Autodesk Inventor part; units mm, degrees
ref_plane "YZ Plane" through (0, 0, 0) normal (1, 0, 0) x (0, 1, 0)
ref_plane "XZ Plane" through (0, 0, 0) normal (0, 1, 0) x (-1, 0, 0)
ref_plane "XY Plane" through (0, 0, 0) normal (0, 0, 1) x (1, 0, 0)
sketch "Sketch1" plane through (0, 0, 0) normal (0, 0, 1) x (1, 0, 0)
  circle A0 centre (0, 0) radius 10.75
  dimension "d0" = 21.5
extrude "Extrusion1" add sketch "Sketch1" along normal blind 48
sketch "Sketch2" plane through (0, 0, 48) normal (0, 0, 1) x (1, 0, 0)
  circle A0 centre (0, 0) radius 10.75
  circle A1 centre (0, 0) radius 5
  dimension "d3" = 10
extrude "Extrusion2" cut sketch "Sketch2" against normal blind 45
chamfer "Chamfer1" distance 0.5 angle 45 1 edges at (-5, 0, 48)
fillet "Fillet1" radius 0.5 1 edges at (-5, 0, 3)
sketch "Sketch3" plane through (0, 0, 0) normal (0, 1, 0) x (-1, 0, 0)
  line L0 (-4.5, 48) -> (4.5, 48)
  line L1 (5, 47.5) -> (-5, 47.5)
  line L2 (-5, 3.5) -> (5, 3.5)
  circle A0 centre (0, 42) radius 2
  point P0 (0, 0)
  dimension "d10" = 4
  dimension "d11" = 6
extrude "Extrusion3" cut sketch "Sketch3" along normal mid plane 15
properties part number "EIXO DAS ENGRENAGENS(11)" material "Carbon Steel"
Check sheet for the modelled part. Datum: model origin and axes. Units: mm. A direction names the side the tool comes from. Give positions to 0.01 mm unless a question says otherwise; leave off trailing zeros. Loops run counter-clockwise (first coordinate to the right, second up) from the corner with the lowest first, then second, coordinate; pieces in that order, holes last. Notation, with made-up numbers: M -1,75.25 L 39,75.25 A16 cw 39,87.25 Z; hole C 21,85.5 d8. An arc over 180 degrees is marked long. Use a Markdown table: item, result. Add a question column.
Q1. Sectioned sample at D-D, the plane z = 15. Record the cut outline in (x, y).
Q2. Sectioned sample at B-B, the plane y = 0. Record the cut outline in (x, z).
Q3. Scan lines: line 1 along X through (y, z) = (-0.25, 42); line 2 along Z through (x, y) = (0, -1.5); line 3 along Z through (x, y) = (4.75, 7.5). Record each from-to range of solid material in increasing order. Write a range as [from, to].
Q4. Sectioned sample at A-A, the plane x = 0. Record the cut outline in (y, z).
Q5. Go/stop test with flat-tipped pins: pin 1 (3 mm diameter, centred on y = 1.5, z = 33.5, fed in from +X); pin 2 (8 mm diameter, centred on x = 7, z = 19.5, fed in from +Y); pin 3 (5 mm diameter, centred on x = 0, z = 42, fed in from +Y); pin 4 (2 mm diameter, centred on x = -7.5, z = 18, fed in from -Y). Record where each tip stops, or that it passes through.
Q6. Tool access check on faces 4 (the flat face through (0, 0, 0)), 5 (the flat face through (-3, 5, 3)). Record the directions out of +Z, -Z, +X, -X, +Y, -Y that give a thin tool (end or side, any length) a straight path to the whole face; none if there is none.
Q7. Mould release check, pull along X, two halves, no side actions. Record for faces 1 (the cylindrical face through (4.77, 1.5, 25.81)), 2 (the cylindrical face through (-0.923, -0.07, 43.774)), 3 (the flat face through (0, 0, 48)): pulls with the +X half, pulls with the -X half, needs draft (parallel to the pull), parting line crosses it, or undercut.
Q8. Sectioned sample at C-C, the plane z = 42. Record the cut outline in (x, y).
Verdict:
| question | item | result |
|---|---|---|
| 1 | outline | C 0,0 d10 |
| 2 | outline | M -10.75,0 L 10.75,0 L 10.75,3 L 5.5,3 A0.5 cw 5,3.5 L 5,47.5 L 4.5,48 L -4.5,48 L -5,47.5 L -5,3.5 A0.5 cw -5.5,3 L -10.75,3 Z; hole C 0,42 d4 |
| 3 | line 1 | [-4.99, -2], [2, 4.99] |
| 3 | line 2 | [0, 40], [44, 48] |
| 3 | line 3 | [0, 3] |
| 4 | outline | M -10.75,0 L 10.75,0 L 10.75,3 L 5.5,3 A0.5 cw 5,3.5 L 5,40 L -5,40 L -5,3.5 A0.5 cw -5.5,3 L -10.75,3 Z; M -5,44 L 5,44 L 5,47.5 L 4.5,48 L -4.5,48 L -5,47.5 Z |
| 5 | pin 1 | x = 5 |
| 5 | pin 2 | y = 4 |
| 5 | pin 3 | y = 5 |
| 5 | pin 4 | through |
| 6 | face 4 | -Z, +X, -X, +Y, -Y |
| 6 | face 5 | +Z |
| 7 | face 1 | parting line crosses it |
| 7 | face 2 | undercut |
| 7 | face 3 | needs draft |
| 8 | outline | M -2,-4.58 L -2,4.58 A5 ccw Z; M 2,-4.58 A5 ccw 2,4.58 Z |
